Design review of the part built by this model. Coordinates are the model's own, in mm. Face numbers are marked on the shaded views. Give positions to 0.01 mm unless a question says otherwise; leave off trailing zeros. Order: outer loops, then holes, each group sorted by start corner. A loop starts at its lowest first (then second) coordinate and runs counter-clockwise, first axis right, second up.
Autodesk Inventor part; units mm, degrees
ref_plane "YZ Plane" through (0, 0, 0) normal (1, 0, 0) x (0, 1, 0)
ref_plane "XZ Plane" through (0, 0, 0) normal (0, 1, 0) x (-1, 0, 0)
ref_plane "XY Plane" through (0, 0, 0) normal (0, 0, 1) x (1, 0, 0)
sketch "Sketch1" plane through (0, 0, 0) normal (1, 0, 0) x (0, 1, 0)
  line L0 (41.284, -14.8819) -> (64.684, -14.8819)
  line L1 (64.684, -13.8819) -> (41.284, -13.8819)
  line L2 (67.684, -8.5819) -> (70.484, -8.5819)
  line L3 (70.484, -8.5819) -> (70.484, -7.5819)
  line L4 (70.484, -7.5819) -> (67.684, -7.5819)
  line L5 (-1817770.1114, -20.3632) -> (-1817770.1114, -8.5819)
  line L6 (38.284, -7.5819) -> (35.484, -7.5819)
  line L7 (35.484, -7.5819) -> (35.484, -8.5819)
  line L8 (35.484, -8.5819) -> (38.284, -8.5819)
  line L9 (40.284, -9.5819) -> (40.284, -12.8819)
  arc A0 (67.684, -8.5819) -> (66.684, -9.5819) centre (67.684, -9.5819) ccw
  arc A1 (64.684, -13.8819) -> (65.684, -12.8819) centre (64.684, -12.8819) ccw
  arc A2 (40.284, -12.8819) -> (41.284, -13.8819) centre (41.284, -12.8819) ccw
  arc A3 (39.284, -9.5819) -> (38.284, -8.5819) centre (38.284, -9.5819) ccw
  arc A4 (40.284, -9.5819) -> (38.284, -7.5819) centre (38.284, -9.5819) ccw
  arc A5 (39.284, -12.8819) -> (41.284, -14.8819) centre (41.284, -12.8819) ccw
  line L10 (39.284, -9.5819) -> (39.284, -12.8819)
  arc A6 (67.684, -7.5819) -> (65.684, -9.5819) centre (67.684, -9.5819) ccw
  arc A7 (64.684, -14.8819) -> (66.684, -12.8819) centre (64.684, -12.8819) ccw
  line L11 (66.684, -9.5819) -> (66.684, -12.8819)
  line L12 (65.684, -9.5819) -> (65.684, -12.8819)
  line L13 (52.984, -4.8951) -> (52.984, -40.6352) construction
  line L14 (-285.558, -25.9225) -> (179.442, -25.9225)
  line L15 (179.442, -25.9225) -> (179.442, -22.9225)
  line L16 (-285.558, -22.9225) -> (179.442, -22.9225)
  line L17 (-285.558, -25.9225) -> (-285.558, -22.9225)
  point P0 (0, 0)
  point P1 (40.284, -11.2319)
  dimension "d0" = 1
  dimension "d1" = 1
  dimension "d5" = 35
  dimension "d8" = 7.3
  dimension "d9" = 1
  dimension "d10" = 1
  dimension "d11" = 2
  dimension "d12" = 2
  dimension "d13" = 12.7
  dimension "d15" = 12.7
  dimension "d16" = 4.8
  dimension "d17" = 4.8
  dimension "d20" = 1
  dimension "d21" = 1
  dimension "d22" = 2
extrude "Extrusion1" add sketch "Sketch1" along normal blind 300 contours A5 L10 A3 L8 L7 L6 A4 L9 A2 L1 A1 L12 A6 L4 L3 L2 A0 L11 A7 L0
sketch "Sketch2" plane through (0, 41.284, -13.8819) normal (0, 0, 1) x (1, 0, 0)
  line L0 (3.6, 11.7) -> (21.6, 11.7) construction
  line L1 (6.8, 8.5) -> (18.4, 8.5)
  line L2 (18.4, 14.9) -> (6.8, 14.9)
  arc A0 (6.8, 14.9) -> (6.8, 8.5) centre (6.8, 11.7) ccw
  arc A1 (18.4, 8.5) -> (18.4, 14.9) centre (18.4, 11.7) ccw
  line L3 (0, 29.2) -> (300, 29.2)
  line L4 (0, -5.8) -> (300, -5.8)
  line L5 (0, 23.4) -> (0, 0)
  arc A2 (31.8, 14.9) -> (31.8, 8.5) centre (31.8, 11.7) ccw
  line L6 (31.8, 8.5) -> (43.4, 8.5)
  arc A3 (43.4, 8.5) -> (43.4, 14.9) centre (43.4, 11.7) ccw
  line L7 (43.4, 14.9) -> (31.8, 14.9)
  arc A4 (56.8, 14.9) -> (56.8, 8.5) centre (56.8, 11.7) ccw
  line L8 (56.8, 8.5) -> (68.4, 8.5)
  arc A5 (68.4, 8.5) -> (68.4, 14.9) centre (68.4, 11.7) ccw
  line L9 (68.4, 14.9) -> (56.8, 14.9)
  arc A6 (81.8, 14.9) -> (81.8, 8.5) centre (81.8, 11.7) ccw
  line L10 (81.8, 8.5) -> (93.4, 8.5)
  arc A7 (93.4, 8.5) -> (93.4, 14.9) centre (93.4, 11.7) ccw
  line L11 (93.4, 14.9) -> (81.8, 14.9)
  arc A8 (106.8, 14.9) -> (106.8, 8.5) centre (106.8, 11.7) ccw
  line L12 (106.8, 8.5) -> (118.4, 8.5)
  arc A9 (118.4, 8.5) -> (118.4, 14.9) centre (118.4, 11.7) ccw
  line L13 (118.4, 14.9) -> (106.8, 14.9)
  arc A10 (131.8, 14.9) -> (131.8, 8.5) centre (131.8, 11.7) ccw
  line L14 (131.8, 8.5) -> (143.4, 8.5)
  arc A11 (143.4, 8.5) -> (143.4, 14.9) centre (143.4, 11.7) ccw
  line L15 (143.4, 14.9) -> (131.8, 14.9)
  arc A12 (156.8, 14.9) -> (156.8, 8.5) centre (156.8, 11.7) ccw
  line L16 (156.8, 8.5) -> (168.4, 8.5)
  arc A13 (168.4, 8.5) -> (168.4, 14.9) centre (168.4, 11.7) ccw
  line L17 (168.4, 14.9) -> (156.8, 14.9)
  arc A14 (181.8, 14.9) -> (181.8, 8.5) centre (181.8, 11.7) ccw
  line L18 (181.8, 8.5) -> (193.4, 8.5)
  arc A15 (193.4, 8.5) -> (193.4, 14.9) centre (193.4, 11.7) ccw
  line L19 (193.4, 14.9) -> (181.8, 14.9)
  line L20 (0, 0) -> (300, 0)
  line L21 (0, 24.4) -> (300, 24.4)
  line L22 (0, -1) -> (300, -1)
  arc A16 (206.8, 14.9) -> (206.8, 8.5) centre (206.8, 11.7) ccw
  line L23 (218.4, 14.9) -> (206.8, 14.9)
  arc A17 (218.4, 8.5) -> (218.4, 14.9) centre (218.4, 11.7) ccw
  line L24 (206.8, 8.5) -> (218.4, 8.5)
  arc A18 (231.8, 14.9) -> (231.8, 8.5) centre (231.8, 11.7) ccw
  line L25 (243.4, 14.9) -> (231.8, 14.9)
  arc A19 (243.4, 8.5) -> (243.4, 14.9) centre (243.4, 11.7) ccw
  line L26 (231.8, 8.5) -> (243.4, 8.5)
  arc A20 (256.8, 14.9) -> (256.8, 8.5) centre (256.8, 11.7) ccw
  line L27 (268.4, 14.9) -> (256.8, 14.9)
  arc A21 (268.4, 8.5) -> (268.4, 14.9) centre (268.4, 11.7) ccw
  line L28 (256.8, 8.5) -> (268.4, 8.5)
  arc A22 (281.8, 14.9) -> (281.8, 8.5) centre (281.8, 11.7) ccw
  line L29 (293.4, 14.9) -> (281.8, 14.9)
  arc A23 (293.4, 8.5) -> (293.4, 14.9) centre (293.4, 11.7) ccw
  line L30 (281.8, 8.5) -> (293.4, 8.5)
  point P0 (0, -41.284)
  point P1 (12.6, 11.7)
  point P2 (28.6, 11.7)
  point P3 (46.6, 11.7)
  point P4 (53.6, 11.7)
  point P5 (71.6, 11.7)
  point P6 (78.6, 11.7)
  point P7 (96.6, 11.7)
  point P8 (103.6, 11.7)
  point P9 (121.6, 11.7)
  point P10 (128.6, 11.7)
  point P11 (146.6, 11.7)
  point P12 (153.6, 11.7)
  point P13 (171.6, 11.7)
  point P14 (178.6, 11.7)
  point P15 (196.6, 11.7)
  point P16 (28.6, 11.7)
  point P17 (203.6, 11.7)
  point P18 (221.6, 11.7)
  point P19 (228.6, 11.7)
  point P20 (246.6, 11.7)
  point P21 (253.6, 11.7)
  point P22 (271.6, 11.7)
  point P23 (278.6, 11.7)
  point P24 (296.6, 11.7)
  dimension "d26" = 18
  dimension "d33" = 25
  dimension "d46" = 3.6
  dimension "d47" = 17.5
  dimension "d48" = 17.5
  dimension "d51" = 25
extrude "Extrusion2" cut sketch "Sketch2" against normal blind 25
sketch "Sketch3" plane through (0, 41.284, -13.8819) normal (0, 0, 1) x (1, 0, 0)
  line L0 (140, 34.2) -> (302, 34.2)
  line L1 (302, 34.2) -> (302, -10.8)
  line L2 (302, -10.8) -> (140, -10.8)
  line L3 (140, -10.8) -> (140, 34.2)
  line L4 (0, 23.4) -> (0, 0)
  line L5 (300, 23.4) -> (300, 0)
  line L6 (0, -5.8) -> (300, -5.8)
  line L7 (0, 29.2) -> (300, 29.2)
  point P0 (0, -41.284)
  dimension "d56" = 140
  dimension "d57" = 2
  dimension "d58" = 5
  dimension "d59" = 5
extrude "Extrusion3" cut sketch "Sketch3" along normal through all both and the other way through all
equation "\"d39\" = d33"
properties part number "DIN-rail-short"
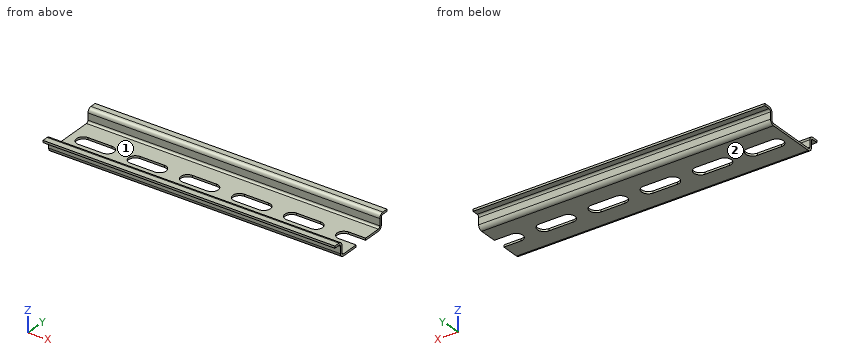
1. Draft analysis for pull direction Y (two halves, no side actions). For the marked faces 1 and 2, state which applies: pulls with the +Y half, pulls with the -Y half, needs draft (parallel to the pull), parting line crosses it, or undercut.
Recorded:
face 1: undercut
face 2: needs draft
2. For pin 1 (2 mm diameter, centred on x = 88, y = 69, fed in from -Z); pin 2 (7 mm diameter, centred on x = 65, y = 55.5, fed in from +Z); pin 3 (0.5 mm diameter, centred on x = 15.5, z = -14.5, fed in from -Y); pin 4 (1 mm diameter, centred on y = 58, z = -13.5, fed in from -X), all flat-tipped, find the tip position at first contact; note any pin that passes through.
Recorded:
pin 1: stops at z = -8.58
pin 2: stops at z = -13.88
pin 3: stops at y = 39.83
pin 4: stops at x = 0
3. Take a section at B-B (z = -11). State the section outline as (x, y) points.
Recorded:
outline: (0, 39.28) - (140, 39.28) - (140, 40.28) - (0, 40.28) - close; (0, 65.68) - (140, 65.68) - (140, 66.68) - (0, 66.68) - close
4. For line 1 along Y through (x, z) = (70.5, -11.75); line 2 along Z through (x, y) = (57, 47.5); line 3 along Z through (x, y) = (58, 37), list the stretches that pass through material, from the lowest coordinate up.
Recorded:
line 1: y = 39.28 to 40.28, 65.68 to 66.68
line 2: z = -14.88 to -13.88
line 3: z = -8.58 to -7.58
5. Take a section at C-C (y = 54.5). State the section outline as (x, z) points.
Recorded:
outline: (0, -14.88) - (3.98, -14.88) - (3.98, -13.88) - (0, -13.88) - close; (21.22, -14.88) - (28.98, -14.88) - (28.98, -13.88) - (21.22, -13.88) - close; (46.22, -14.88) - (53.98, -14.88) - (53.98, -13.88) - (46.22, -13.88) - close; (71.22, -14.88) - (78.98, -14.88) - (78.98, -13.88) - (71.22, -13.88) - close; (96.22, -14.88) - (103.98, -14.88) - (103.98, -13.88) - (96.22, -13.88) - close; (121.22, -14.88) - (128.98, -14.88) - (128.98, -13.88) - (121.22, -13.88) - close
6. Take a section at A-A (x = 59.5). State the section outline as (y, z) points.
Recorded:
outline: (35.48, -8.58) - (38.28, -8.58) arc R1 cw to (39.28, -9.58) - (39.28, -12.88) arc R2 ccw to (41.28, -14.88) - (49.78, -14.88) - (49.78, -13.88) - (41.28, -13.88) arc R1 cw to (40.28, -12.88) - (40.28, -9.58) arc R2 ccw to (38.28, -7.58) - (35.48, -7.58) - close; (56.18, -14.88) - (64.68, -14.88) arc R2 ccw to (66.68, -12.88) - (66.68, -9.58) arc R1 cw to (67.68, -8.58) - (70.48, -8.58) - (70.48, -7.58) - (67.68, -7.58) arc R2 ccw to (65.68, -9.58) - (65.68, -12.88) arc R1 cw to (64.68, -13.88) - (56.18, -13.88) - close
7. Take a section at D-D (y = 62.5). State the section outline as (x, z) points.
Recorded:
outline: (0, -14.88) - (140, -14.88) - (140, -13.88) - (0, -13.88) - close
